from build123d import *

# Parameters (mm, degrees)
BOSS_EXTRUDE1_DEPTH = 19.05
SKETCH2_R           = 3.1115
BOSS_EXTRUDE3_DEPTH = 5.00888
CUT_EXTRUDE1_DEPTH  = 37.525855062
SKETCH3_R           = 6.35
CUT_EXTRUDE2_DEPTH  = 40.436271203
SKETCH5_W           = 10.16
SKETCH5_H           = 10.16
CUT_EXTRUDE3_DEPTH  = 40.436271203


with BuildPart() as part:
    # Sketch1 → Boss-Extrude1 (new body)
    with BuildSketch(Plane.XY):
        with BuildLine():
            Line((-16.764, 10.535978608), (-13.649989304, 13.649989304))
            ThreePointArc((-13.649989304, 13.649989304), (-11.72846788, 15.33256199), (-9.60163475, 16.746731805))
            Line((-9.60163475, 16.746731805), (-0.635, 16.746731805))
            Line((-0.635, 16.746731805), (-0.635, 11.666731805))
            ThreePointArc((-0.635, 11.666731805), (0, -11.684), (0.635, 11.666731805))
            Line((0.635, 11.666731805), (0.635, 16.746731805))
            Line((0.635, 16.746731805), (9.60163475, 16.746731805))
            ThreePointArc((9.60163475, 16.746731805), (11.72846788, 15.33256199), (13.649989304, 13.649989304))
            Line((13.649989304, 13.649989304), (16.764, 10.535978608))
            Line((16.764, 10.535978608), (16.764, -19.304))
            Line((16.764, -19.304), (-16.764, -19.304))
            Line((-16.764, -19.304), (-16.764, 10.535978608))
        make_face()
    extrude(amount=BOSS_EXTRUDE1_DEPTH)

    # Sketch2 → Boss-Extrude3 (add)
    with BuildSketch(Plane.ZY.offset(-0.635)):
        with BuildLine():
            Line((19.05, 16.746731805), (0, 16.746731805))
            ThreePointArc((0, 16.746731805), (9.525, 26.271731805), (19.05, 16.746731805))
        make_face()
        with Locations(Location((9.525, 20.048731805, 0), (0, 0, 270))):
            Circle(SKETCH2_R, mode=Mode.SUBTRACT)
    boss_extrude3 = extrude(amount=-BOSS_EXTRUDE3_DEPTH)

    # Mirror7: Boss-Extrude3 across plane
    add(boss_extrude3.mirror(Plane(origin=(0, 0, 0), x_dir=(0, 0, 1), z_dir=(1, 0, 0))))

    # Sketch4 → Cut-Extrude1 (cut, through all)
    with BuildSketch(Plane(origin=(0, 0, 0), x_dir=(-1, 0, 0), z_dir=(0, 0, -1))):
        with BuildLine():
            Line((-16.141246803, 11.158731805), (-16.141246803, 17.710333674))
            Line((-16.141246803, 17.710333674), (-5.64388, 16.746731805))
            add(Edge.make_bspline(
                [(-5.64388, 16.746731805), (-11.711664831, 15.588313777), (-16.141246803, 11.158731805)],
                knots=[0, 0, 0, 1, 1, 1], degree=2))
        make_face()
        with BuildLine():
            Line((16.141246803, 17.710333674), (5.64388, 16.746731805))
            add(Edge.make_bspline(
                [(5.64388, 16.746731805), (11.711664831, 15.588313777), (16.141246803, 11.158731805)],
                knots=[0, 0, 0, 1, 1, 1], degree=2))
            Line((16.141246803, 11.158731805), (16.141246803, 17.710333674))
        make_face()
    extrude(amount=-CUT_EXTRUDE1_DEPTH, mode=Mode.SUBTRACT)

    # Sketch3 → Cut-Extrude2 (cut, through all)
    with BuildSketch(Plane.ZY.offset(5.64388)):
        with Locations((9.525, 20.048731805)):
            Circle(SKETCH3_R)
    extrude(amount=CUT_EXTRUDE2_DEPTH, mode=Mode.SUBTRACT)

    # Sketch5 → Cut-Extrude3 (cut, through all)
    with BuildSketch(Plane(origin=(5.64388, 0, 0), x_dir=(0, 0, -1), z_dir=(1, 0, 0))):
        with Locations((-9.525, 20.048731805)):
            Rectangle(SKETCH5_W, SKETCH5_H)
    extrude(amount=CUT_EXTRUDE3_DEPTH, mode=Mode.SUBTRACT)


solid = part.part
For this review, take the finished solid that the model builds, in its own axes (mm). A direction names the side the tool comes from. Round coordinates to 2 decimals unless told otherwise and drop trailing zeros. Write each loop counter-clockwise with the first axis right and the second up, starting at its lowest first coordinate (ties: lowest second). Pieces come first, ordered by that corner, then holes. Notation, with made-up numbers: (31, 46.5) -> (66, 46.5) arc R21 ccw to (66, 68.5) -> close; hole circle Ø5 at (-1, 39). An arc over 180 degrees is marked (long way). Use CSV: the item, a comma, the result in double quotes.
(1) Clearance check with flat-ended pins moving along their axes: P1, Ø10, axis at y = 22, z = 8, coming from the -X side; P2, Ø3.5, axis at y = 21, z = 5.5, coming from the +X side; P3, Ø3.5, axis at y = 20.05, z = 9.52, coming from the -X side; P4, Ø7.5, axis at y = 16, z = 7, coming from the +X side. State where each tip first meets the part, or that it passes through.
Computed values:
P1,"x = -5.64"
P2,"x = 5.64"
P3,"through"
P4,"x = 14.97"
(2) For faces 1 (the face through (-5.644, 17, 12)), 2 (the face through (8, -9, 19.05)), 3 (the face through (-0.635, 17, 8)), 4 (the face through (8, 14.969, 10)), 5 (the face through (-16.764, -5, 9)), list the 3-axis set-ups (+Z, -Z, +X, -X, +Y, -Y) from which the entire face can be reached by the end or side of a thin tool; tool diameter is ignored.
Computed values:
face 1,"-X, +Y"
face 2,"+Z, +X, -X, +Y, -Y"
face 3,"+Z, -Z, +Y"
face 4,"+X, +Y"
face 5,"+Z, -Z, -X, +Y, -Y"
(3) To check wall thickness, follow L1, parallel to Y at x = -1.5, z = 10.25; L2, parallel to Y at x = 5, z = 6.75; L3, parallel to Y at x = -0.5, z = 6.5. State the ranges of each line that lie inside material, in increasing order. Write a range as [from, to].
Computed values:
L1,"[-19.3, -11.59], [11.59, 17.02], [23.07, 26.24]"
L2,"[-19.3, -10.56], [10.56, 18.64], [21.46, 25.86]"
L3,"[-19.3, -11.67]"
(4) Consider section B-B, the plane x = -3.5. Give the number of separate pieces and of enclosed holes in the cut face, plus the area to 3 significant figures.
Computed values:
separate pieces,"2"
enclosed holes,"1"
area,"374 mm²"
(5) Consider section A-A, the plane y = 0. Give the boundary of the cut face in (x, z).
Computed values:
outline,"(-16.76, 0) -> (-11.68, 0) -> (-11.68, 19.05) -> (-16.76, 19.05) -> close; (11.68, 0) -> (16.76, 0) -> (16.76, 19.05) -> (11.68, 19.05) -> close"
(6) Draft analysis for pull direction X (two halves, no side actions). For faces 6 (the face through (-0.505, -11.673, 9.392)), 7 (the face through (0.635, 17, 8)), 8 (the face through (-3.1, 26.27, 9.32)), 9 (the face through (16.764, -4, 9)), state which applies: +X half, -X half, draft (parallel to the pull), parting line (faces both ways), or undercut.
Computed values:
face 6,"undercut"
face 7,"undercut"
face 8,"draft"
face 9,"+X half"
